from build123d import *

# Parameters (mm, degrees)
F1_DEPTH = 2
F2_DEPTH = 21
F3_R     = 2
F4_W     = 2
F4_H     = 5
F4_W_2   = 8
F4_H_2   = 0.55
F4_H_3   = 0.1
F5_DEPTH = 2.2
F6_R     = 0.5
F7_DEPTH = 2.9
F8_DEPTH = 1.25


with BuildPart() as f1:
    # F0 (on Top) → F1 (new body)
    with BuildSketch(Plane.XY):
        with BuildLine():
            Line((-44.875, -29.75), (44.875, -29.75))
            ThreePointArc((44.875, -29.75), (48.4105339059, -28.2855339059), (49.875, -24.75))
            Line((49.875, -24.75), (49.875, 24.75))
            ThreePointArc((49.875, 24.75), (48.4105339059, 28.2855339059), (44.875, 29.75))
            Line((44.875, 29.75), (-44.875, 29.75))
            ThreePointArc((-44.875, 29.75), (-48.4105339059, 28.2855339059), (-49.875, 24.75))
            Line((-49.875, 24.75), (-49.875, -24.75))
            ThreePointArc((-49.875, -24.75), (-48.4105339059, -28.2855339059), (-44.875, -29.75))
        make_face()
        with BuildLine():
            ThreePointArc((47.875, -25.25), (47.142766953, -27.017766953), (45.375, -27.75))
            Line((45.375, -27.75), (-45.375, -27.75))
            ThreePointArc((-45.375, -27.75), (-47.142766953, -27.017766953), (-47.875, -25.25))
            Line((-47.875, -25.25), (-47.875, 25.25))
            ThreePointArc((-47.875, 25.25), (-47.142766953, 27.017766953), (-45.375, 27.75))
            Line((-45.375, 27.75), (45.375, 27.75))
            ThreePointArc((45.375, 27.75), (47.142766953, 27.017766953), (47.875, 25.25))
            Line((47.875, 25.25), (47.875, -25.25))
        make_face(mode=Mode.SUBTRACT)
        with BuildLine():
            Line((-45.375, -27.75), (45.375, -27.75))
            ThreePointArc((45.375, -27.75), (47.142766953, -27.017766953), (47.875, -25.25))
            Line((47.875, -25.25), (47.875, 25.25))
            ThreePointArc((47.875, 25.25), (47.142766953, 27.017766953), (45.375, 27.75))
            Line((45.375, 27.75), (-45.375, 27.75))
            ThreePointArc((-45.375, 27.75), (-47.142766953, 27.017766953), (-47.875, 25.25))
            Line((-47.875, 25.25), (-47.875, -25.25))
            ThreePointArc((-47.875, -25.25), (-47.142766953, -27.017766953), (-45.375, -27.75))
        make_face()
    extrude(amount=F1_DEPTH)

    # F0 (on Top) → F2 (join)
    with BuildSketch(Plane.XY):
        with BuildLine():
            Line((-44.875, -29.75), (44.875, -29.75))
            ThreePointArc((44.875, -29.75), (48.4105339059, -28.2855339059), (49.875, -24.75))
            Line((49.875, -24.75), (49.875, 24.75))
            ThreePointArc((49.875, 24.75), (48.4105339059, 28.2855339059), (44.875, 29.75))
            Line((44.875, 29.75), (-44.875, 29.75))
            ThreePointArc((-44.875, 29.75), (-48.4105339059, 28.2855339059), (-49.875, 24.75))
            Line((-49.875, 24.75), (-49.875, -24.75))
            ThreePointArc((-49.875, -24.75), (-48.4105339059, -28.2855339059), (-44.875, -29.75))
        make_face()
        with BuildLine():
            ThreePointArc((47.875, -25.25), (47.142766953, -27.017766953), (45.375, -27.75))
            Line((45.375, -27.75), (-45.375, -27.75))
            ThreePointArc((-45.375, -27.75), (-47.142766953, -27.017766953), (-47.875, -25.25))
            Line((-47.875, -25.25), (-47.875, 25.25))
            ThreePointArc((-47.875, 25.25), (-47.142766953, 27.017766953), (-45.375, 27.75))
            Line((-45.375, 27.75), (45.375, 27.75))
            ThreePointArc((45.375, 27.75), (47.142766953, 27.017766953), (47.875, 25.25))
            Line((47.875, 25.25), (47.875, -25.25))
        make_face(mode=Mode.SUBTRACT)
    extrude(amount=F2_DEPTH)

    # F3
    f3_edges = [f1.edges().sort_by_distance(p)[0] for p in [
        (0, -29.75, 0),
        (-48.410534, -28.285534, 0),
        (-49.875, 0, 0),
        (-48.410534, 28.285534, 0),
        (0, 29.75, 0),
        (48.410534, 28.285534, 0),
        (49.875, 0, 0),
        (48.410534, -28.285534, 0),
    ]]
    fillet(f3_edges, radius=F3_R)

    # F4 (on face) → F5 (cut)
    with BuildSketch(Plane.XY.offset(21)):
        with Locations((-48.875, -18.75)):
            Rectangle(F4_W, F4_H)
        with Locations((-48.875, 18.75)):
            Rectangle(F4_W, F4_H)
        with Locations((-33.625, 28.125)):
            Rectangle(F4_W_2, F4_H_2)
        with Locations((-33.625, 27.8)):
            Rectangle(F4_W_2, F4_H_3)
        with Locations((33.625, 28.125)):
            Rectangle(F4_W_2, F4_H_2)
        with Locations((33.625, 27.8)):
            Rectangle(F4_W_2, F4_H_3)
    extrude(amount=-F5_DEPTH, mode=Mode.SUBTRACT)

    # F6
    f6_edges = [f1.edges().sort_by_distance(p)[0] for p in [
        (47.142767, 27.017767, 2),
        (47.875, 0, 2),
        (47.142767, -27.017767, 2),
        (0, -27.75, 2),
        (-47.142767, -27.017767, 2),
        (-47.875, 0, 2),
        (-47.142767, 27.017767, 2),
        (0, 27.75, 2),
    ]]
    fillet(f6_edges, radius=F6_R)

    # F4 (on face) → F7 (cut)
    with BuildSketch(Plane.XY.offset(21)):
        with Locations((-33.625, -28.125)):
            Rectangle(F4_W_2, F4_H_2)
        with Locations((-33.625, -27.8)):
            Rectangle(F4_W_2, F4_H_3)
        with Locations((33.625, -27.8)):
            Rectangle(F4_W_2, F4_H_3)
        with Locations((33.625, -28.125)):
            Rectangle(F4_W_2, F4_H_2)
    extrude(amount=-F7_DEPTH, mode=Mode.SUBTRACT)

    # F4 (on face) → F8 (join)
    with BuildSketch(Plane.XY.offset(21)):
        with Locations((33.625, 28.125)):
            Rectangle(F4_W_2, F4_H_2)
        with Locations((-33.625, 28.125)):
            Rectangle(F4_W_2, F4_H_2)
        with Locations((-33.625, -28.125)):
            Rectangle(F4_W_2, F4_H_2)
        with Locations((33.625, -28.125)):
            Rectangle(F4_W_2, F4_H_2)
    extrude(amount=-F8_DEPTH)


solid = f1.part
Geometry: final body of the model. Coordinates: model frame, mm. A direction names the side the tool comes from. Round coordinates to 2 decimals unless told otherwise and drop trailing zeros. Loops run counter-clockwise (first coordinate to the right, second up) from the corner with the lowest first, then second, coordinate; pieces in that order, holes last. Notation, with made-up numbers: (57.25, 30.5) - (93.25, 30.5) arc R15 ccw to (93.25, 34.5) - close; hole circle Ø6 at (43.5, 52). An arc over 180 degrees is marked (long way). Write each question's results on one line, items separated by ' | '. Start each with the question number.
1) Mould query, pull axis X, two halves, no side actions, for faces 4 (the face through (-48.371, 28.324, 11.367)), 5 (the face through (-49, -16.25, 20)), 6 (the face through (47.16, -27, 11.62)). Classes: released by +X, released by -X, zero draft, split by the parting line, or undercut.
2) Cut plane C-C on x = -8. Return loops of the section in (y, z), then the cut area to 3 significant figures.
3) First-contact query: P1, Ø2, axis at x = 21.5, y = 10, coming from the +Z side; P2, Ø1.6, axis at x = -49.5, z = 20, coming from the +Y side; P3, Ø0.5, axis at y = -28, z = 19, coming from the -X side (3 decimals). Flat tips, straight axial feed; report the tip coordinate or a pass-through.
4) Line query: probe 1 along X at (y, z) = (23.5, 4.5) (3 decimals); probe 2 along Y at (x, z) = (-45, 17.25). Output: solid intervals per line, ascending. Write a range as [from, to].
5) Access query for faces 1 (the face through (-49, -21.25, 20)), 2 (the face through (-47.875, 0, 12)), 3 (the face through (-49.875, 0, 11)). Directions: +Z, -Z, +X, -X, +Y, -Y. A direction counts if a zero-diameter tool reaches every point of the face in a straight line with its end or side. Return the directions, or none.
6) Cut plane D-D on x = 31. Return loops of the section in (y, z), then the cut area to 3 significant figures.
7) Cut plane B-B on y = 0.5. Return loops of the section in (x, z) (3 decimals).
8) Cut plane A-A on z = 7.5. Return loops of the section in (x, y) (3 decimals), then the cut area to 3 significant figures.
Verdict:
1) face 4: released by -X | face 5: zero draft | face 6: undercut
2) outline: (-29.75, 2) arc R2 ccw to (-27.75, 0) - (27.75, 0) arc R2 ccw to (29.75, 2) - (29.75, 21) - (27.75, 21) - (27.75, 2.5) arc R0.5 cw to (27.25, 2) - (-27.25, 2) arc R0.5 cw to (-27.75, 2.5) - (-27.75, 21) - (-29.75, 21) - close | area: 193 mm2
3) P1: stops at z = 2 | P2: stops at y = 27.97 | P3: stops at x = -48.875
4) probe 1: x = [-49.875, -47.875], [47.875, 49.875] | probe 2: y = [-29.75, -27.75], [27.75, 29.75]
5) face 1: +Z, -X | face 2: +Z | face 3: +Z, -Z, -X, +Y, -Y
6) outline: (-29.75, 2) arc R2 ccw to (-27.75, 0) - (27.75, 0) arc R2 ccw to (29.75, 2) - (29.75, 21) - (27.85, 21) - (27.85, 19.75) - (28.4, 19.75) - (28.4, 18.8) - (27.75, 18.8) - (27.75, 2.5) arc R0.5 cw to (27.25, 2) - (-27.25, 2) arc R0.5 cw to (-27.75, 2.5) - (-27.75, 18.1) - (-28.4, 18.1) - (-28.4, 19.75) - (-27.85, 19.75) - (-27.85, 21) - (-29.75, 21) - close | area: 191 mm2
7) outline: (-49.875, 2) arc R2 ccw to (-47.875, 0) - (47.875, 0) arc R2 ccw to (49.875, 2) - (49.875, 21) - (47.875, 21) - (47.875, 2.5) arc R0.5 cw to (47.375, 2) - (-47.375, 2) arc R0.5 cw to (-47.875, 2.5) - (-47.875, 21) - (-49.875, 21) - close
8) outline: (-49.875, -24.75) arc R5 ccw to (-44.875, -29.75) - (44.875, -29.75) arc R5 ccw to (49.875, -24.75) - (49.875, 24.75) arc R5 ccw to (44.875, 29.75) - (-44.875, 29.75) arc R5 ccw to (-49.875, 24.75) - close; hole (-47.875, -25.25) arc R2.5 ccw to (-45.375, -27.75) - (45.375, -27.75) arc R2.5 ccw to (47.875, -25.25) - (47.875, 25.25) arc R2.5 ccw to (45.375, 27.75) - (-45.375, 27.75) arc R2.5 ccw to (-47.875, 25.25) - close | area: 605 mm2
